Answer from the drawing. Dimensions are ordinates in mm from the lowest x, y and z of the part. A direction names the side the tool comes from. Round coordinates to 2 decimals unless told otherwise and drop trailing zeros. Loops run counter-clockwise (first coordinate to the right, second up) from the corner with the lowest first, then second, coordinate; pieces in that order, holes last. Notation, with made-up numbers: M 20.5,22.25 L 52.5,22.25 A16 cw 52.5,28.25 Z; hole C -7.75,53 d6. An arc over 180 degrees is marked long. One line per item, written item: value.
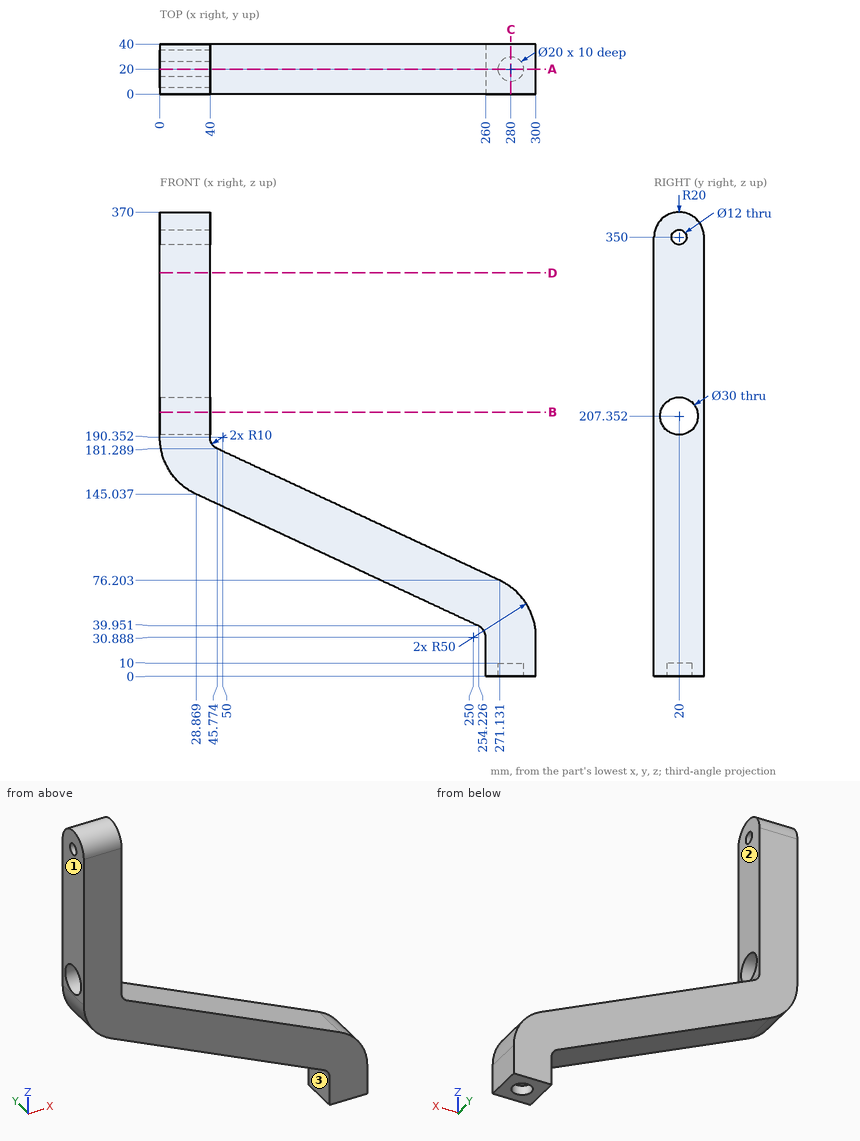
1) Find section C-C (x = 280). Give the vertices of the cut face in (y, z), then the cut area to 3 significant figures.
Check values:
outline: M 0,0 L 10,0 L 10,10 L 30,10 L 30,0 L 40,0 L 40,70.89 L 0,70.89 Z
area: 2,640 mm2
2) Find section B-B (z = 210.5). Give the vertices of the cut face in (x, y).
Check values:
outline: M 0,0 L 40,0 L 40,5.33 L 0,5.33 Z; M 0,34.67 L 40,34.67 L 40,40 L 0,40 Z
3) Each of these flat-tipped pins is pushed along its axis until it touches: pin 1 (4 mm diameter, centred on x = 232.5, y = 30, fed in from -Z); pin 2 (1.5 mm diameter, centred on x = 56.5, y = 23.5, fed in from -Z); pin 3 (15.5 mm diameter, centred on y = 16, z = 15.5, fed in from -X). Where does it stop, or does it pass through?
Check values:
pin 1: z = 49.15
pin 2: z = 131.8
pin 3: x = 260
4) Find section A-A (y = 20). Give the vertices of the cut face in (x, z), then the cut area to 3 significant figures.
Check values:
outline: M 0,190.35 A50 ccw 28.87,145.04 L 254.23,39.95 A10 cw 260,30.89 L 260,0 L 270,0 L 270,10 L 290,10 L 290,0 L 300,0 L 300,30.89 A50 ccw 271.13,76.2 L 45.77,181.29 A10 cw 40,190.35 L 40,192.35 L 0,192.35 Z; M 0,222.35 L 40,222.35 L 40,344 L 0,344 Z; M 0,356 L 40,356 L 40,370 L 0,370 Z
area: 19,200 mm2
5) For the marked faces 1, 2 and 3, determine the directions among +Z, -Z, +X, -X, +Y, -Y from which every point of the face is accessible in a straight line to the end or side of a thin tool.
Check values:
face 1: +Z, -Z, -X, +Y, -Y
face 2: +Z, +X, +Y, -Y
face 3: -Z, -X, +Y, -Y
6) Find the intervals of material crossed by probe 1 along Y at (x, z) = (18, 350); probe 2 along Y at (x, z) = (280, 7); probe 3 along X at (y, z) = (26.5, 340), in increasing order. Write a range as from..to.
Check values:
probe 1: 0..14, 26..40
probe 2: 0..10, 30..40
probe 3: 0..40
7) Find section D-D (z = 321.5). Give the vertices of the cut face in (x, y), then the cut area to 3 significant figures.
Check values:
outline: M 0,0 L 40,0 L 40,40 L 0,40 Z
area: 1,600 mm2
